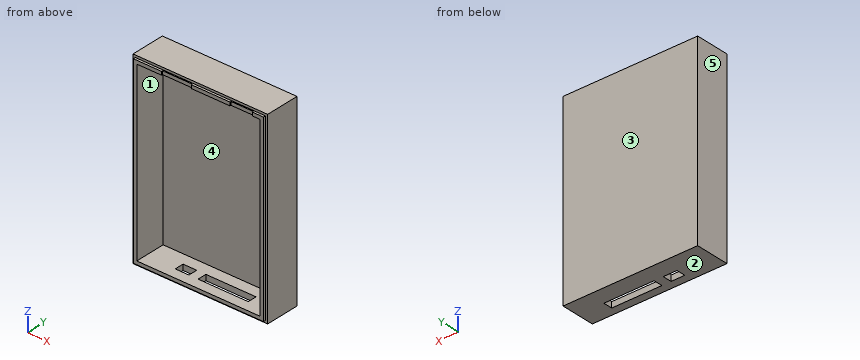
Autodesk Inventor part; units mm, degrees
ref_plane "Work Plane1" through (0, 2.5, 0) normal (0, -1, 0) x (1, 0, 0)
ref_plane "YZ Plane" through (0, 0, 0) normal (1, 0, 0) x (0, 1, 0)
ref_plane "XZ Plane" through (0, 0, 0) normal (0, 1, 0) x (-1, 0, 0)
sketch "Sketch1" plane through (0, 0, 0) normal (0, 1, 0) x (-1, 0, 0)
  line L0 (0, 0) -> (59, 0)
  line L1 (59, 0) -> (59, -82)
  line L2 (59, -82) -> (0, -82)
  line L3 (0, -82) -> (0, 0)
  dimension "d0" = 82
  dimension "d1" = 59
extrude "Extrusion1" add sketch "Sketch1" along normal blind 32
ref_plane "Work Plane1" through (0, 2.5, 0) normal (0, -1, 0) x (1, 0, 0)
sketch "Sketch2" plane through (0, 2.5, 0) normal (0, -1, 0) x (1, 0, 0)
  line L0 (-2.5, -2.5) -> (-56.5, -2.5)
  line L1 (-56.5, -2.5) -> (-56.5, -79.5)
  line L2 (-56.5, -79.5) -> (-2.5, -79.5)
  line L3 (-2.5, -79.5) -> (-2.5, -2.5)
  line L4 (0, 0) -> (0, -82)
  line L5 (-59, 0) -> (0, 0)
  line L6 (-59, -82) -> (-59, 0)
  line L7 (0, -82) -> (-59, -82)
  dimension "d5" = 2.5
  dimension "d6" = 2.5
  dimension "d7" = 2.5
  dimension "d8" = 2.5
extrude "Extrusion2" cut sketch "Sketch2" against normal blind 27 contours L3 L2 L1 L0
sketch "Sketch3" plane through (0, 2.5, 0) normal (0, -1, 0) x (1, 0, 0)
  line L0 (-3, -3) -> (-56, -3) construction
  line L1 (-56, -3) -> (-56, -79) construction
  line L2 (-56, -79) -> (-3, -79) construction
  line L3 (-3, -79) -> (-3, -3) construction
  line L4 (-2.5, -2.5) -> (-2.5, -79.5)
  line L5 (-56.5, -2.5) -> (-2.5, -2.5)
  line L6 (-56.5, -79.5) -> (-56.5, -2.5)
  line L7 (-2.5, -79.5) -> (-56.5, -79.5)
  circle A0 centre (-53.8, -24.59) radius 1.65
  circle A1 centre (-5.54, -23.32) radius 1.65
  circle A2 centre (-38.56, -75.39) radius 1.65
  circle A3 centre (-10.62, -75.39) radius 1.65
  point P0 (0, 0)
  dimension "d11" = 0.5
  dimension "d12" = 0.5
  dimension "d13" = 0.5
  dimension "d14" = 0.5
  dimension "d15" = 3.3
  dimension "d16" = 20.32
  dimension "d17" = 2.54
  dimension "d18" = 7.62
  dimension "d19" = 72.39
  dimension "d20" = 21.59
  dimension "d22" = 50.8
  dimension "d23" = 35.56
  dimension "d24" = 72.39
extrude "Extrusion3" cut sketch "Sketch3" along normal blind 27 contours A0 | A1 | A2 | A3
sketch "Sketch4" plane through (-59, 0, 0) normal (0, 0, 1) x (1, 0, 0)
  line L0 (13.4, 5.6) -> (26.4, 5.6)
  line L1 (26.4, 5.6) -> (26.4, 16.5)
  line L2 (26.4, 16.5) -> (13.4, 16.5)
  line L3 (13.4, 16.5) -> (13.4, 5.6)
  line L4 (43.3, 5.6) -> (53.2, 5.6)
  line L5 (53.2, 5.6) -> (53.2, 16.5)
  line L6 (53.2, 16.5) -> (43.3, 16.5)
  line L7 (43.3, 16.5) -> (43.3, 5.6)
  line L8 (56.5, 2.5) -> (2.5, 2.5)
  line L9 (2.5, 2.5) -> (2.5, 29.5)
  line L10 (56.5, 2.5) -> (56.5, 29.5)
  point P0 (59, 0)
  dimension "d27" = 13
  dimension "d28" = 10.9
  dimension "d29" = 9.9
  dimension "d31" = 14
  dimension "d32" = 10.9
  dimension "d33" = 3.3
extrude "Extrusion4" cut sketch "Sketch4" against normal blind 5
sketch "Sketch5" plane through (0, 0, -82) normal (0, 0, -1) x (-1, 0, 0)
  line L0 (11.5, 24.5) -> (33.5, 24.5)
  line L1 (33.5, 24.5) -> (33.5, 20.5)
  line L2 (33.5, 20.5) -> (11.5, 20.5)
  line L3 (11.5, 20.5) -> (11.5, 24.5)
  line L4 (37.5, 24.5) -> (43.5, 24.5)
  line L5 (43.5, 24.5) -> (43.5, 20.5)
  line L6 (43.5, 20.5) -> (37.5, 20.5)
  line L7 (37.5, 20.5) -> (37.5, 24.5)
  line L8 (56.5, 2.5) -> (2.5, 2.5)
  line L9 (2.5, 2.5) -> (2.5, 29.5)
  point P0 (0, 0)
  dimension "d36" = 22
  dimension "d37" = 4
  dimension "d38" = 4
  dimension "d39" = 22
  dimension "d40" = 9
  dimension "d41" = 6
  dimension "d42" = 4
extrude "Extrusion5" cut sketch "Sketch5" against normal blind 5
sketch "Sketch6" plane through (-59, 0, -82) normal (-1, 0, 0) x (0, 0, 1)
  circle A0 centre (57.41, 6) radius 1.6
  line L0 (79.5, 2.5) -> (79.5, 29.5)
  line L1 (82, 0) -> (0, 0)
  dimension "d45" = 3.2
  dimension "d46" = 22.09
  dimension "d47" = 6
sketch "Sketch7" plane through (0, 0, 0) normal (1, 0, 0) x (0, 0, -1)
  circle A0 centre (23.32, 6) radius 1.6
  line L0 (82, 0) -> (0, 0)
  line L1 (2.5, 2.5) -> (2.5, 29.5)
  dimension "d48" = 6
  dimension "d49" = 20.82
  dimension "d50" = 3.2
sketch "Sketch8" plane through (0, 0, -82) normal (0, 0, -1) x (-1, 0, 0)
  circle A0 centre (10.62, 6) radius 1.6
  circle A1 centre (38.56, 6) radius 1.6
  line L0 (59, 0) -> (0, 0)
  line L1 (2.5, 2.5) -> (2.5, 29.5)
  dimension "d51" = 3.2
  dimension "d52" = 3.2
  dimension "d53" = 6
  dimension "d54" = 6
  dimension "d55" = 8.12
  dimension "d56" = 36.06
extrude "Extrusion6" cut sketch "Sketch6" against normal blind 5
extrude "Extrusion7" cut sketch "Sketch7" against normal blind 5
extrude "Extrusion8" cut sketch "Sketch8" against normal blind 5
sketch "Sketch9" plane through (-59, 0, 0) normal (0, 0, 1) x (1, 0, 0)
  line L0 (-2.1645, 16) -> (66.4826, 16)
  line L1 (59, 0) -> (0, 0)
  dimension "d63" = 16
split body "Split1" sketch "Sketch9" result one side removed curves L0 removed pieces at (-32.4383, 0.5, -41.3152)
sketch "Sketch10" plane through (-59, 16, -82) normal (0, -1, 0) x (1, 0, 0)
  line L0 (0, 82) -> (59, 82)
  line L1 (59, 82) -> (59, 0)
  line L2 (0, 82) -> (59, 82)
  line L3 (59, 82) -> (59, 0)
  line L4 (59, 0) -> (0, 0)
  line L5 (0, 0) -> (0, 82)
  line L6 (58, 1) -> (1, 1)
  line L7 (1, 1) -> (1, 81)
  line L8 (1, 81) -> (58, 81)
  line L9 (58, 81) -> (58, 1)
  dimension "d64" = 1
  dimension "d65" = 1
  dimension "d66" = 1
  dimension "d67" = 1
extrude "Extrusion9" cut sketch "Sketch10" against normal blind 1
properties part number "Arduino_Box_Upper"
Part model, mm, in its own coordinate system. Face numbers are marked on the shaded views. A direction names the side the tool comes from. Coordinates: 2 decimals unless noted, no trailing zeros. Order: outer loops, then holes, each group sorted by start corner. A loop starts at its lowest first (then second) coordinate and runs counter-clockwise, first axis right, second up. Notation, with made-up numbers: M 87.25,14.25 L 97.25,14.25 A14 cw 97.25,28.25 Z; hole C 80.25,59.5 d1. An arc over 180 degrees is marked long. One line per question, with ' | ' between items.
Q1. Slice it at A-A (x = -27.5). Give the cut face in (y, z), and give its area (4 significant figures).
A:
outline: M 16,-81 L 17,-81 L 17,-82 L 20.5,-82 L 20.5,-79.5 L 16,-79.5 Z; M 16,-2.5 L 29.5,-2.5 L 29.5,-79.5 L 24.5,-79.5 L 24.5,-82 L 32,-82 L 32,0 L 17,0 L 17,-1 L 16,-1 Z | area: 260.5 mm^2
Q2. Slice it at C-C (y = 22.25). Give the cut face in (x, z).
A:
outline: M -59,-82 L -43.5,-82 L -43.5,-79.5 L -56.5,-79.5 L -56.5,-2.5 L -2.5,-2.5 L -2.5,-79.5 L -11.5,-79.5 L -11.5,-82 L 0,-82 L 0,0 L -59,0 Z; M -37.5,-82 L -33.5,-82 L -33.5,-79.5 L -37.5,-79.5 Z
Q3. Slice it at D-D (x = -9). Give the cut face in (y, z), and give its area (3 significant figures).
A:
outline: M 16,-81 L 17,-81 L 17,-82 L 32,-82 L 32,0 L 17,0 L 17,-1 L 16.5,-1 L 16.5,-2.5 L 29.5,-2.5 L 29.5,-79.5 L 16,-79.5 Z | area: 270 mm^2
Q4. Slice it at B-B (y = 28.25). Give the cut face in (x, z), and give its area (3 significant figures).
A:
outline: M -59,-82 L 0,-82 L 0,0 L -59,0 Z; hole M -56.5,-79.5 L -2.5,-79.5 L -2.5,-2.5 L -56.5,-2.5 Z | area: 680 mm^2
Q5. Pin check, flat tip, straight feed: P1, Ø1.2, axis at x = -36, z = -1.5, coming from the -Y side. Stop position of the tip, or through.
A:
P1: stops at y = 16.5
Q6. 3-axis set-ups, long thin cutter, end or side, ignore diameter. For the marked faces 4 and 5: which of +Z, -Z, +X, -X, +Y, -Y reach the whole face in a straight line?
A:
face 4: -Y | face 5: +Z, -Z, -X, +Y, -Y
Q7. Two-plate mould, pull along Z, no slides. Class the marked faces 1, 2 and 3: +Z half, -Z half, draft (parallel to the pull), parting line (faces both ways), or undercut.
A:
face 1: undercut | face 2: -Z half | face 3: draft
Q8. Drill centre lines: line 1 (X direction, y = 23, z = -46); line 2 (Z direction, x = -16, y = 28); line 3 (Y direction, x = -35.5, z = -26). Where is each one in solid material? Low to high.
A:
line 1: x = -59 to -56.5, -2.5 to 0 | line 2: z = -82 to -79.5, -2.5 to 0 | line 3: y = 29.5 to 32
